Could you check a few things on this model? Use its own coordinates, in mm. Face numbers are marked on the shaded views. Give positions to 0.01 mm unless a question says otherwise; leave off trailing zeros. Loops run counter-clockwise (first coordinate to the right, second up) from the corner with the lowest first, then second, coordinate; pieces in that order, holes last. Notation, with made-up numbers: M -17.5,12.25 L 25.5,12.25 A16 ccw 25.5,38.25 Z; hole C 0.25,-27 d5. An arc over 180 degrees is marked long. Answer in a Markdown table with one row per item. Add a question column.
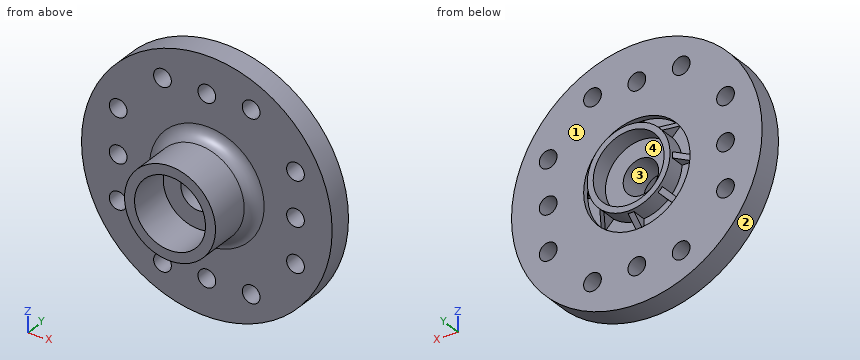
```python
from build123d import *

# Parameters (mm, degrees)
SKETCH1_R           = 10.6
BOSS_EXTRUDE1_DEPTH = 2
SKETCH2_R           = 0.75
CUT_EXTRUDE2_DEPTH  = 3
CIRPATTERN1_COUNT   = 4
SKETCH3_R           = 3.85
BOSS_EXTRUDE2_DEPTH = 4.5
SKETCH4_R           = 3
CUT_EXTRUDE3_DEPTH  = 3.5
SKETCH5_R           = 1.5
CUT_EXTRUDE4_DEPTH  = 4
FILLET1_R           = 1
SKETCH6_R           = 4.5
CUT_EXTRUDE5_DEPTH  = 0.5
SKETCH7_R           = 3.5
SKETCH7_R_2         = 3
BOSS_EXTRUDE3_DEPTH = 1.5
BOSS_EXTRUDE4_DEPTH = 0.25
CIRPATTERN2_COUNT   = 8


with BuildPart() as part:
    # Sketch1 → Boss-Extrude1 (new body)
    with BuildSketch(Plane(origin=(0, 0, 0), x_dir=(1, 0, 0), z_dir=(0, 1, 0))):
        Circle(SKETCH1_R)
    extrude(amount=BOSS_EXTRUDE1_DEPTH)

    # Sketch2 → Cut-Extrude2 (cut, through all)
    with BuildSketch(Plane(origin=(0, 0, 0), x_dir=(1, 0, 0), z_dir=(0, 1, 0))):
        with Locations((-3.75, 7.5)):
            Circle(SKETCH2_R)
        with Locations((3.75, 7.5)):
            Circle(SKETCH2_R)
        with Locations((0, 7.5)):
            Circle(SKETCH2_R)
    cut_extrude2 = extrude(amount=CUT_EXTRUDE2_DEPTH, mode=Mode.SUBTRACT)

    # CirPattern1: Cut-Extrude2 ×4 about axis
    cirpattern1_axis = Axis((0, 0, 0), (0, 1, 0))
    for i in range(1, CIRPATTERN1_COUNT):
        add(cut_extrude2.rotate(cirpattern1_axis, i * 360 / CIRPATTERN1_COUNT), mode=Mode.SUBTRACT)

    # Sketch3 → Boss-Extrude2 (add)
    with BuildSketch(Plane.XZ):
        Circle(SKETCH3_R)
    extrude(amount=BOSS_EXTRUDE2_DEPTH)

    # Sketch4 → Cut-Extrude3 (cut)
    with BuildSketch(Plane.XZ.offset(4.5)):
        Circle(SKETCH4_R)
    extrude(amount=-CUT_EXTRUDE3_DEPTH, mode=Mode.SUBTRACT)

    # Sketch5 → Cut-Extrude4 (cut, through all)
    with BuildSketch(Plane.XZ.offset(1)):
        Circle(SKETCH5_R)
    extrude(amount=-CUT_EXTRUDE4_DEPTH, mode=Mode.SUBTRACT)

    # Fillet1
    fillet1_edges = [part.edges().sort_by_distance(p)[0] for p in [
        (-3.85, 0, 0),
    ]]
    fillet(fillet1_edges, radius=FILLET1_R)

    # Sketch6 → Cut-Extrude5 (cut)
    with BuildSketch(Plane(origin=(0, 2, 0), x_dir=(1, 0, 0), z_dir=(0, 1, 0))):
        Circle(SKETCH6_R)
    extrude(amount=-CUT_EXTRUDE5_DEPTH, mode=Mode.SUBTRACT)

    # Sketch7 → Boss-Extrude3 (add)
    with BuildSketch(Plane(origin=(0, 1.5, 0), x_dir=(1, 0, 0), z_dir=(0, 1, 0))):
        Circle(SKETCH7_R)
        Circle(SKETCH7_R_2, mode=Mode.SUBTRACT)
    extrude(amount=BOSS_EXTRUDE3_DEPTH)

    # Sketch8 → Boss-Extrude4 (add, symmetric)
    with BuildSketch(Plane(origin=(0, 0, 0), x_dir=(0, 0, -1), z_dir=(1, 0, 0))):
        Polygon((-4.5, 1.5), (-3, 1.5), (-3, 3), (-3.25, 3), align=None)
    boss_extrude4 = extrude(amount=BOSS_EXTRUDE4_DEPTH, both=True)

    # CirPattern2: Boss-Extrude4 ×8 about axis
    cirpattern2_axis = Axis((0, 0, 0), (0, 1, 0))
    for i in range(1, CIRPATTERN2_COUNT):
        add(boss_extrude4.rotate(cirpattern2_axis, i * 360 / CIRPATTERN2_COUNT))


solid = part.part
```
Item 1: If we mould it in two halves opening along X, with no side actions, what happens to the marked faces 1, 2, 3 and 4? For each: +X half, -X half, draft (parallel to the pull), parting line (faces both ways), or undercut.
Item 2: For P1, Ø0.5, axis at y = 2, z = 3.5, coming from the -X side; P2, Ø6, axis at x = -1, z = -7.5, coming from the -Y side; P3, Ø3, axis at x = -1, z = 1, coming from the -Y side, each with a flat end and sliding along its axis, tell me the tip position at first contact or that it passes through.
Item 3: Suppose I cut it at D-D (x = 0). Give the number of separate pieces and of enclosed holes in the cut face, then the cut area to 3 significant figures.
Item 4: I need wall thicknesses on L1, parallel to Z at x = 0, y = 0.05; L2, parallel to Z at x = 8, y = 1.25; L3, parallel to X at y = 0.55, z = 7.5. Which ranges of each line are inside material? Lowest first, please.
Item 5: Suppose I cut it at A-A (x = -7.5). List the corners of the cut face in (y, z) for me.
Item 6: Suppose I cut it at B-B (z = -7.5). List the corners of the cut face in (x, y) for me, then the cut area to 3 significant figures.
Item 7: Suppose I cut it at C-C (y = -3.75). List the corners of the cut face in (x, z) for me.
Values found:
| question | item | result |
|---|---|---|
| 1 | face 1 | draft |
| 1 | face 2 | parting line |
| 1 | face 3 | undercut |
| 1 | face 4 | undercut |
| 2 | P1 | x = -10.09 |
| 2 | P2 | y = -0.04 |
| 2 | P3 | y = -1 |
| 3 | separate pieces | 4 |
| 3 | enclosed holes | 0 |
| 3 | area | 41.2 mm² |
| 4 | L1 | -10.6 to -8.25, -6.75 to -1.5, 1.5 to 6.75, 8.25 to 10.6 |
| 4 | L2 | -6.95 to -4.31, -3.19 to -0.56, 0.56 to 3.19, 4.31 to 6.95 |
| 4 | L3 | -7.49 to -4.5, -3 to -0.75, 0.75 to 3, 4.5 to 7.49 |
| 5 | outline | M 0,-7.49 L 2,-7.49 L 2,-4.5 L 0,-4.5 Z; M 0,-3 L 2,-3 L 2,-0.75 L 0,-0.75 Z; M 0,0.75 L 2,0.75 L 2,3 L 0,3 Z; M 0,4.5 L 2,4.5 L 2,7.49 L 0,7.49 Z |
| 6 | outline | M -7.49,0 L -4.5,0 L -4.5,2 L -7.49,2 Z; M -3,0 L -0.75,0 L -0.75,2 L -3,2 Z; M 0.75,0 L 3,0 L 3,2 L 0.75,2 Z; M 4.5,0 L 7.49,0 L 7.49,2 L 4.5,2 Z |
| 6 | area | 21.0 mm² |
| 7 | outline | C 0,0 d7.7; hole C 0,0 d6 |
